For this review, use the dimensioned drawing (mm, ordinates from the lowest corner) and the shaded views. Coordinates: 2 decimals unless noted, no trailing zeros. Loops run counter-clockwise (first coordinate to the right, second up) from the corner with the lowest first, then second, coordinate; pieces in that order, holes last. Notation, with made-up numbers: (32, 22.25) -> (70, 22.25) arc R22 ccw to (70, 36.25) -> close; hole circle Ø5 at (43, -6). An arc over 180 degrees is marked (long way). Answer as a JSON object with one key per item and string values.
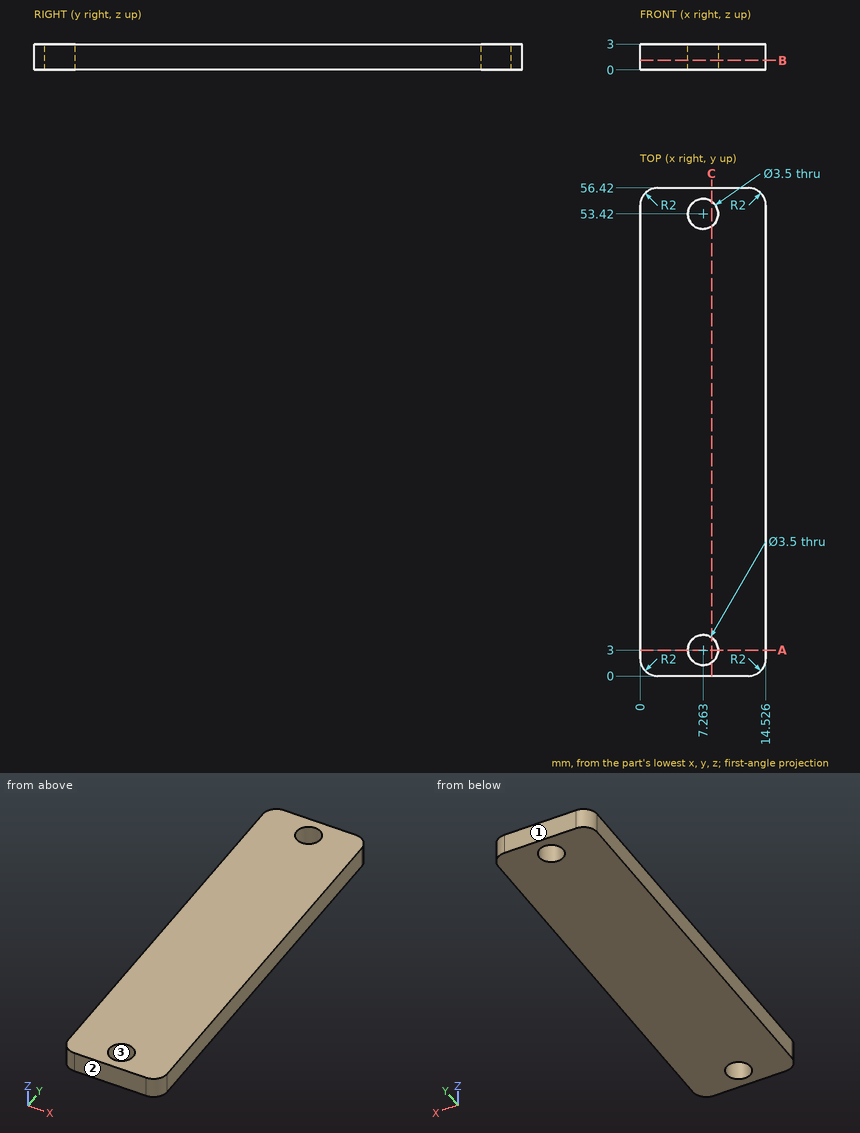
1) Add section A-A, the plane y = 3. Give the boundary of the cut face in (x, z).
Completed:
{"outline": "(0, 0) -> (5.51, 0) -> (5.51, 3) -> (0, 3) -> close; (9.01, 0) -> (14.53, 0) -> (14.53, 3) -> (9.01, 3) -> close"}
2) Add section B-B, the plane z = 1.1. Give the boundary of the cut face in (x, y).
Completed:
{"outline": "(0, 2) arc R2 ccw to (2, 0) -> (12.53, 0) arc R2 ccw to (14.53, 2) -> (14.53, 54.42) arc R2 ccw to (12.53, 56.42) -> (2, 56.42) arc R2 ccw to (0, 54.42) -> close; hole circle Ø3.5 at (7.26, 3); hole circle Ø3.5 at (7.26, 53.42)"}
3) The part is to be moulded in two halves that separate along Y. For the marked faces 1, 2 and 3, say which applies: pulls with the +Y half, pulls with the -Y half, needs draft (parallel to the pull), parting line crosses it, or undercut.
Completed:
{"face 1": "pulls with the +Y half", "face 2": "pulls with the -Y half", "face 3": "undercut"}
4) Wall thickness on probe 1 along X at (y, z) = (3, 2.15); probe 2 along Y at (x, z) = (8, 0.85); probe 3 along Y at (x, z) = (8.5, 2.6): over which ranges is each line inside the solid? List them lowest first.
Completed:
{"probe 1": "0 to 5.51, 9.01 to 14.53", "probe 2": "0 to 1.41, 4.59 to 51.83, 55.01 to 56.42", "probe 3": "0 to 1.76, 4.24 to 52.18, 54.66 to 56.42"}
5) Add section C-C, the plane x = 8.25. Give the boundary of the cut face in (y, z).
Completed:
{"outline": "(0, 0) -> (1.55, 0) -> (1.55, 3) -> (0, 3) -> close; (4.45, 0) -> (51.97, 0) -> (51.97, 3) -> (4.45, 3) -> close; (54.87, 0) -> (56.42, 0) -> (56.42, 3) -> (54.87, 3) -> close"}
